from build123d import *

# Parameters (mm, degrees)
SKETCH_1_R      = 5
SKETCH_1_R_2    = 2.5
EXTRUDE_1_DEPTH = 4
SKETCH_2_W      = 1.193229727
SKETCH_2_H      = 0.975939513


with BuildPart() as part:
    # 草图1 → 凸台-拉伸1 (new body)
    with BuildSketch(Plane(origin=(0, 0, 0), x_dir=(1, 0, 0), z_dir=(0, 1, 0))):
        with Locations(Location((0, 0, 0), (0, 0, 270))):
            Circle(SKETCH_1_R)
        with Locations(Location((0, 0, 0), (0, 0, 270))):
            Circle(SKETCH_1_R_2, mode=Mode.SUBTRACT)
    extrude(amount=EXTRUDE_1_DEPTH)

    # 草图2 → 切除-旋转1 (revolve, cut)
    with BuildSketch(Plane.XY, mode=Mode.PRIVATE) as cut_revolve_1_sk:
        with Locations((-4.403385136, 1.883358194)):
            Rectangle(SKETCH_2_W, SKETCH_2_H)
    revolve(cut_revolve_1_sk.sketch.rotate(Axis((0, 4, 0), (0, -1, 0)), 270), axis=Axis((0, 4, 0), (0, -1, 0)), mode=Mode.SUBTRACT)


solid = part.part
For this review, take the finished solid that the model builds, in its own axes (mm). A direction names the side the tool comes from. Give positions to 0.01 mm unless a question says otherwise; leave off trailing zeros. Order: outer loops, then holes, each group sorted by start corner. A loop starts at its lowest first (then second) coordinate and runs counter-clockwise, first axis right, second up. Notation, with made-up numbers: (-35, 20) -> (3, 20) arc R15 ccw to (3, 33) -> close; hole circle Ø8 at (-36, -31). An arc over 180 degrees is marked (long way). Write item = value, one per line.
1) We need section D-D, the plane z = -2.75. Give the boundary of the cut face in (x, y).
Findings:
outline = (-4.18, 0) -> (4.18, 0) -> (4.18, 1.4) -> (2.63, 1.4) -> (2.63, 2.37) -> (4.18, 2.37) -> (4.18, 4) -> (-4.18, 4) -> (-4.18, 2.37) -> (-2.63, 2.37) -> (-2.63, 1.4) -> (-4.18, 1.4) -> close
2) Draft analysis for pull direction X (two halves, no side actions). For faces 3 (the face through (-2.44, 1.97, -0.54)), 4 (the face through (-1.14, 1.89, 3.63)), 5 (the face through (4, 2.371, -1)), state which applies: pulls with the +X half, pulls with the -X half, needs draft (parallel to the pull), parting line crosses it, or undercut.
Findings:
face_3 = undercut
face_4 = parting line crosses it
face_5 = needs draft
3) To check wall thickness, follow L1, parallel to X at y = 2.25, z = 0; L2, parallel to X at y = 3.1, z = 0; L3, parallel to Y at x = -4, z = -1.25. State the ranges of each line that lie inside material, in increasing order. Write a range as from..to.
Findings:
L1 = -3.81..-2.5, 2.5..3.81
L2 = -5..-2.5, 2.5..5
L3 = 0..1.4, 2.37..4
4) Insertion check: pin 1 (2 mm diameter, centred on y = 2.5, z = 3, fed in from +X). The pin has a flat end and moves straight along its axis. Give the tip position at first contact, or say it passes through.
Findings:
pin_1 = 4.58
5) We need section B-B, the plane x = 0. Give the boundary of the cut face in (y, z).
Findings:
outline = (0, -5) -> (1.4, -5) -> (1.4, -3.81) -> (2.37, -3.81) -> (2.37, -5) -> (4, -5) -> (4, -2.5) -> (0, -2.5) -> close; (0, 2.5) -> (4, 2.5) -> (4, 5) -> (2.37, 5) -> (2.37, 3.81) -> (1.4, 3.81) -> (1.4, 5) -> (0, 5) -> close
6) We need section C-C, the plane y = 0.9. Give the boundary of the cut face in (x, z).
Findings:
outline = circle Ø10 at (0, 0); hole circle Ø5 at (0, 0)
7) We need section A-A, the plane z = 0. Give the boundary of the cut face in (x, y).
Findings:
outline = (-5, 0) -> (-2.5, 0) -> (-2.5, 4) -> (-5, 4) -> (-5, 2.37) -> (-3.81, 2.37) -> (-3.81, 1.4) -> (-5, 1.4) -> close; (2.5, 0) -> (5, 0) -> (5, 1.4) -> (3.81, 1.4) -> (3.81, 2.37) -> (5, 2.37) -> (5, 4) -> (2.5, 4) -> close
8) For faces 1 (the face through (4, 1.395, -1)), 2 (the face through (-2, 0, 2)), list the 3-axis set-ups (+Z, -Z, +X, -X, +Y, -Y) from which the entire face can be reached by the end or side of a thin tool; tool diameter is ignored.
Findings:
face_1 = none
face_2 = +Z, -Z, +X, -X, -Y
